from build123d import *

# Parameters (mm, degrees)
SKETCH1_R               = 3.048
BOSS_EXTRUDE1_DEPTH     = 41.91
CUT_EXTRUDE1_START      = -7.62
CUT_EXTRUDE1_DEPTH      = 7.62
CUT_EXTRUDE2_DEPTH      = 43.216756152
CUT_EXTRUDE2_DEPTH_BACK = 43.216756152
SKETCH3_R               = 1.27
F_6_32_TAPPED_HOLE1_D   = 2.7051


with BuildPart() as part:
    # Sketch1 → Boss-Extrude1 (new body)
    with BuildSketch(Plane.XY):
        Circle(SKETCH1_R)
    extrude(amount=BOSS_EXTRUDE1_DEPTH)

    # Sketch2 → Cut-Extrude1 (cut)
    with BuildSketch(Plane.XY.offset(41.91).offset(CUT_EXTRUDE1_START)):
        with BuildLine():
            ThreePointArc((1.016, 2.873681959), (0.515422831, 3.00410441), (0, 3.048))
            ThreePointArc((0, 3.048), (-0.515422831, 3.00410441), (-1.016, 2.873681959))
            Line((-1.016, 2.873681959), (-1.016, -2.873681959))
            ThreePointArc((-1.016, -2.873681959), (-0.515422831, -3.00410441), (0, -3.048))
            ThreePointArc((0, -3.048), (0.515422831, -3.00410441), (1.016, -2.873681959))
            Line((1.016, -2.873681959), (1.016, 2.873681959))
        make_face()
    extrude(amount=CUT_EXTRUDE1_DEPTH, mode=Mode.SUBTRACT)

    # Sketch3 → Cut-Extrude2 (cut, two sides: drawn at the far end of the back side and taken through both)
    with BuildSketch(Plane(origin=(-1.016, 0, 0), x_dir=(0, 0, -1), z_dir=(1, 0, 0)).offset(-CUT_EXTRUDE2_DEPTH_BACK)):
        with Locations((-38.735, 0)):
            Circle(SKETCH3_R)
    extrude(amount=CUT_EXTRUDE2_DEPTH + CUT_EXTRUDE2_DEPTH_BACK, mode=Mode.SUBTRACT)

    # #6-32 Tapped Hole1 (through all)
    with Locations(Plane(origin=(0, 0, 0), x_dir=(-1, 0, 0), z_dir=(0, 0, -1))):
        with Locations((0, 0), (6.460869533, -0.946768866)):
            Hole(F_6_32_TAPPED_HOLE1_D / 2)


solid = part.part
Can you work these out from the model? Positions are in its coordinate system, mm. A direction names the side the tool comes from. Coordinates: 2 decimals unless noted, no trailing zeros. Loops run counter-clockwise (first coordinate to the right, second up) from the corner with the lowest first, then second, coordinate; pieces in that order, holes last. Notation, with made-up numbers: M -17,31.5 L 11,31.5 A16 ccw 11,52.5 Z; hole C 59,87 d4. An arc over 180 degrees is marked long. Answer as CSV lines item,"result". Start each with the question number.
1. For pin 1 Ø2 at (y, z) = (1.5, 37) entering from -X; pin 2 Ø1 at (y, z) = (2, 40) entering from +X; pin 3 Ø1.5 at (x, z) = (1.5, 35.5) entering from +Y, each with a flat end and sliding along its axis, tell me the tip position at first contact or that it passes through.
2. Suppose I cut it at A-A, the plane y = 0. List the corners of the cut face in (x, z) for me (3 decimals), plus the area to 4 significant figures.
3. Thinking about a two-plate mould opening in Y: for faces 1 (the face through (0, -2, 34.29)), 2 (the face through (2.8, -1.2, 20.7)), 3 (the face through (1.352, -0.014, 40.79)), which applies, +Y half, -Y half, draft (parallel to the pull), parting line (faces both ways), or undercut?
4. Suppose I cut it at D-D, the plane x = -2.5. List the corners of the cut face in (y, z) for me (3 decimals), plus the area to 3 significant figures.
5. For faces 4 (the face through (-1.016, -2, 38)), 5 (the face through (-1.352, 0.014, 40.79)), 6 (the face through (2, 0.1, 40)), which set-ups out of +Z, -Z, +X, -X, +Y, -Y let a thin tool reach every point of the face, with its end or its side?
6. Suppose I cut it at C-C, the plane z = 17.5. List the corners of the cut face in (x, y) for me, plus the area to 3 significant figures.
7. If I drill on probe 1 along Y at (x, z) = (0, 29.5); probe 2 along Z at (x, y) = (1.5, 0) (3 decimals), over which ranges is the centre line in solid material (lowest first)? Write a range as [from, to].
8. Suppose I cut it at B-B, the plane x = 0. List the corners of the cut face in (y, z) for me, plus the area to 3 significant figures.
Output:
1,pin 1,"stops at x = -3.01"
1,pin 2,"stops at x = 2.65"
1,pin 3,"stops at y = 2.87"
2,outline,"M -3.048,0 L -1.353,0 L -1.353,37.465 L -3.048,37.465 Z; M -3.048,40.005 L -1.353,40.005 L -1.353,41.91 L -3.048,41.91 Z; M 1.353,0 L 3.048,0 L 3.048,37.465 L 1.353,37.465 Z; M 1.353,40.005 L 3.048,40.005 L 3.048,41.91 L 1.353,41.91 Z"
2,area,"133.5 mm^2"
3,face 1,"draft"
3,face 2,"parting line"
3,face 3,"undercut"
4,outline,"M -1.744,0 L 1.744,0 L 1.744,41.91 L -1.744,41.91 Z; hole C 0,38.735 d2.54"
4,area,"141 mm^2"
5,face 4,"+Z, +Y, -Y"
5,face 5,"+Z, -Z"
5,face 6,"+X, -X"
6,outline,"C 0,0 d6.1; hole C 0,0 d2.71"
6,area,"23.4 mm^2"
7,probe 1,"y = [-3.05, -1.35], [1.35, 3.05]"
7,probe 2,"z = [0, 37.465], [40.005, 41.91]"
8,outline,"M -3.05,0 L -1.35,0 L -1.35,34.29 L -3.05,34.29 Z; M 1.35,0 L 3.05,0 L 3.05,34.29 L 1.35,34.29 Z"
8,area,"116 mm^2"
